```python
from build123d import *

# Parameters (mm, degrees)
SKETCH_1_R      = 5
SKETCH_1_W      = 41.919872981
SKETCH_1_H      = 10
EXTRUDE_1_DEPTH = 5
FILLET_1_R      = 2
FILLET_2_R      = 2


with BuildPart() as part:
    # 草图1 → 凸台-拉伸1 (new body)
    with BuildSketch(Plane.XY):
        with BuildLine():
            Line((0, 10), (230, 10))
            ThreePointArc((230, 10), (240, 0), (230, -10))
            Line((230, -10), (0, -10))
            ThreePointArc((0, -10), (-10, 0), (0, 10))
        make_face()
        Circle(SKETCH_1_R, mode=Mode.SUBTRACT)
        with Locations((200, 0)):
            Circle(SKETCH_1_R, mode=Mode.SUBTRACT)
        with BuildLine():
            Line((8.660254038, 5), (50.580127019, 5))
            Line((50.580127019, 5), (50.580127019, -5))
            Line((50.580127019, -5), (8.660254038, -5))
            ThreePointArc((8.660254038, -5), (10, 0), (8.660254038, 5))
        make_face(mode=Mode.SUBTRACT)
        with BuildLine():
            Line((208.660254038, 5), (230, 5))
            ThreePointArc((230, 5), (235, 0), (230, -5))
            Line((230, -5), (208.660254038, -5))
            ThreePointArc((208.660254038, -5), (210, 0), (208.660254038, 5))
        make_face(mode=Mode.SUBTRACT)
        with Locations((123.45993649, 0)):
            Rectangle(SKETCH_1_W, SKETCH_1_H, mode=Mode.SUBTRACT)
        with Locations((76.54006351, 0)):
            Rectangle(SKETCH_1_W, SKETCH_1_H, mode=Mode.SUBTRACT)
        with BuildLine():
            Line((149.419872981, -5), (191.339745962, -5))
            ThreePointArc((191.339745962, -5), (190, 0), (191.339745962, 5))
            Line((191.339745962, 5), (149.419872981, 5))
            Line((149.419872981, 5), (149.419872981, -5))
        make_face(mode=Mode.SUBTRACT)
    extrude(amount=EXTRUDE_1_DEPTH)

    # 圆角1
    fillet_1_edges = [part.edges().sort_by_distance(p)[0] for p in [
        (50.580127019, 5, 2.5),
    ]]
    fillet(fillet_1_edges, radius=FILLET_1_R)

    # 圆角2
    fillet_2_edges = [part.edges().sort_by_distance(p)[0] for p in [
        (208.660254038, 5, 2.5),
        (208.660254038, -5, 2.5),
        (144.419872981, 5, 2.5),
        (102.5, 5, 2.5),
        (102.5, -5, 2.5),
        (144.419872981, -5, 2.5),
        (191.339745962, -5, 2.5),
        (191.339745962, 5, 2.5),
        (149.419872981, 5, 2.5),
        (149.419872981, -5, 2.5),
        (8.660254038, 5, 2.5),
        (8.660254038, -5, 2.5),
        (50.580127019, -5, 2.5),
        (97.5, 5, 2.5),
        (55.580127019, 5, 2.5),
        (55.580127019, -5, 2.5),
        (97.5, -5, 2.5),
    ]]
    fillet(fillet_2_edges, radius=FILLET_2_R)


solid = part.part
```
For this review, take the finished solid that the model builds, in its own axes (mm). A direction names the side the tool comes from. Coordinates: 2 decimals unless noted, no trailing zeros. Loops run counter-clockwise (first coordinate to the right, second up) from the corner with the lowest first, then second, coordinate; pieces in that order, holes last.
1. Add section A-A, the plane x = 36. Give the boundary of the cut face in (y, z), then the cut area to 3 significant figures.
2. Add section B-B, the plane y = 0. Count the separate pieces of the cut face and the enclosed holes in it, then the cut area to 3 significant figures.
3. Mouldability with a two-part tool opening along X and no side actions: class faces 3 (the cylindrical face through (240, 0, 2)), 4 (the flat face through (170, 5, 2)), 5 (the flat face through (117, 7, 0)) as +X half, -X half, draft (parallel to the pull), parting line (faces both ways), or undercut.
4. Insertion check: P1, Ø1.5, axis at y = -7.5, z = 1.5, coming from the -X side. The pin has a flat end and moves straight along its axis. Give the tip position at first contact, or say it passes through.
5. For line 1 (Y direction, x = 12, z = 1.85); line 2 (X direction, y = 7.5, z = 2.75); line 3 (X direction, y = 8, z = 2.85), list the stretches that pass through material, from the lowest coordinate up.
6. For faces 1 (the flat face through (117, -10, 2)), 2 (the flat face through (149.42, 0, 2)), list the 3-axis set-ups (+Z, -Z, +X, -X, +Y, -Y) from which the entire face can be reached by the end or side of a thin tool; tool diameter is ignored.
Result:
1. outline: (-10, 0) - (-5, 0) - (-5, 5) - (-10, 5) - close; (5, 0) - (10, 0) - (10, 5) - (5, 5) - close
1. area: 50.0 mm2
2. separate pieces: 8
2. enclosed holes: 0
2. area: 200 mm2
3. face 3: +X half
3. face 4: undercut
3. face 5: draft
4. P1: stops at x = -7.38
5. line 1: y = -10 to -5, 5 to 10
5. line 2: x = -6.61 to 236.61
5. line 3: x = -6 to 236
6. face 1: +Z, -Z, +X, -X, -Y
6. face 2: +Z, -Z
